from build123d import *

# Parameters (mm, degrees)
SALIENTE_EXTRUIR1_DEPTH    = 172
VACIADO2_T                 = -2
SALIENTE_EXTRUIR2_DEPTH    = 30
CORTAR_EXTRUIR2_DEPTH      = 186.698680663
CORTAR_EXTRUIR2_DEPTH_BACK = 186.698680663
CORTAR_EXTRUIR3_DEPTH      = 184.847763109
CORTAR_EXTRUIR3_DEPTH_BACK = 25
CROQUIS8_R                 = 3.75
CORTAR_EXTRUIR4_DEPTH      = 186.698680663
CORTAR_EXTRUIR4_DEPTH_BACK = 186.698680663
CROQUIS9_W                 = 61.645841287
CROQUIS9_H                 = 31
CORTAR_EXTRUIR5_DEPTH      = 158.419820861
CORTAR_EXTRUIR5_DEPTH_BACK = 158.419820861


with BuildPart() as part:
    # Croquis1 → Saliente-Extruir1 (new body)
    with BuildSketch(Plane(origin=(0, 0, 0), x_dir=(1, 0, 0), z_dir=(0, 1, 0))):
        Polygon((27, 0), (-27, 0), (0, 64.58327957), align=None)
    extrude(amount=SALIENTE_EXTRUIR1_DEPTH)

    # Vaciado2
    vaciado2_openings = [part.faces().sort_by_distance(p)[0] for p in [
        (0, 172, -21.527759857),
    ]]
    offset(amount=VACIADO2_T, openings=vaciado2_openings, kind=Kind.INTERSECTION)

    # Croquis6 → Saliente-Extruir2 (add)
    with BuildSketch(Plane.XZ):
        Polygon((-27, 0), (27, 0), (0, -64.58327957), align=None)
    extrude(amount=SALIENTE_EXTRUIR2_DEPTH)

    # Croquis5 → Cortar-Extruir2 (cut, two sides: drawn at the far end of the back side and taken through both)
    with BuildSketch(Plane(origin=(0, 0, 0), x_dir=(0, 0, -1), z_dir=(1, 0, 0)).offset(-CORTAR_EXTRUIR2_DEPTH_BACK)):
        Polygon((4.522801595, 172), (64.58327957, 172), (64.58327957, 0), align=None)
    extrude(amount=CORTAR_EXTRUIR2_DEPTH + CORTAR_EXTRUIR2_DEPTH_BACK, mode=Mode.SUBTRACT)

    # Croquis8 → Cortar-Extruir3 (cut, two sides: drawn at the far end of the back side and taken through both)
    with BuildSketch(Plane(origin=(0, 2, 0), x_dir=(1, 0, 0), z_dir=(0, 1, 0)).offset(-CORTAR_EXTRUIR3_DEPTH_BACK)):
        with Locations(Location((0, 48.787977385, 0), (0, 0, 270))):
            Circle(CROQUIS8_R)
        with Locations(Location((0, 38.787977385, 0), (0, 0, 270))):
            Circle(CROQUIS8_R)
        with Locations(Location((0, 28.787977385, 0), (0, 0, 270))):
            Circle(CROQUIS8_R)
        with Locations(Location((0, 18.787977385, 0), (0, 0, 270))):
            Circle(CROQUIS8_R)
        with Locations(Location((0, 8.787977385, 0), (0, 0, 270))):
            Circle(CROQUIS8_R)
        with Locations(Location((10, 8.787977385, 0), (0, 0, 270))):
            Circle(CROQUIS8_R)
        with Locations(Location((-10, 8.787977385, 0), (0, 0, 270))):
            Circle(CROQUIS8_R)
        with Locations(Location((10, 18.787977385, 0), (0, 0, 270))):
            Circle(CROQUIS8_R)
        with Locations(Location((-10, 18.787977385, 0), (0, 0, 270))):
            Circle(CROQUIS8_R)
        with Locations(Location((8, 28.787977385, 0), (0, 0, 270))):
            Circle(CROQUIS8_R)
        with Locations(Location((-8, 28.787977385, 0), (0, 0, 270))):
            Circle(CROQUIS8_R)
    extrude(amount=CORTAR_EXTRUIR3_DEPTH + CORTAR_EXTRUIR3_DEPTH_BACK, mode=Mode.SUBTRACT)

    # Croquis9 → Cortar-Extruir4 (cut, two sides: drawn at the far end of the back side and taken through both)
    with BuildSketch(Plane(origin=(0, 0, 0), x_dir=(0, 0, -1), z_dir=(1, 0, 0)).offset(-CORTAR_EXTRUIR4_DEPTH_BACK)):
        with Locations((30.822920644, 156.5)):
            Rectangle(CROQUIS9_W, CROQUIS9_H)
    extrude(amount=CORTAR_EXTRUIR4_DEPTH + CORTAR_EXTRUIR4_DEPTH_BACK, mode=Mode.SUBTRACT)

    # Croquis10 → Cortar-Extruir5 (cut, two sides: drawn at the far end of the back side and taken through both)
    with BuildSketch(Plane(origin=(0, 0, 0), x_dir=(0, 0, -1), z_dir=(1, 0, 0)).offset(-CORTAR_EXTRUIR5_DEPTH_BACK)):
        Polygon((0, 141), (64.58327957, 0), (23.73241025, 141), align=None)
    extrude(amount=CORTAR_EXTRUIR5_DEPTH + CORTAR_EXTRUIR5_DEPTH_BACK, mode=Mode.SUBTRACT)


solid = part.part
Can you work these out from the model? Positions are in its coordinate system, mm. A direction names the side the tool comes from. Give positions to 0.01 mm unless a question says otherwise; leave off trailing zeros. Loops run counter-clockwise (first coordinate to the right, second up) from the corner with the lowest first, then second, coordinate; pieces in that order, holes last. Notation, with made-up numbers: (55.5, 71) - (102.5, 71) arc R26 ccw to (102.5, 94) - close; hole circle Ø11 at (27, 48). An arc over 180 degrees is marked (long way). Return JSON: item names as keys, results as strings.
1. I want a section at A-A on x = -8. Please give me the cut outline in (y, z), and give its area (3 significant figures).
Output values:
{"outline": "(-30, -45.45) - (41.78, -45.45) - (53.1, -40.26) - (2, -40.26) - (2, -32.54) - (-23, -32.54) - (-23, -25.04) - (2, -25.04) - (2, -21.96) - (-23, -21.96) - (-23, -15.62) - (2, -15.62) - (2, -11.96) - (-23, -11.96) - (-23, -5.62) - (2, -5.62) - (2, -2) - (136.63, -2) - (141, 0) - (-30, 0) - close", "area": "1,460 mm²"}
2. If I drill on line 1 (Z direction, x = -8, y = -8); line 2 (Z direction, x = -10, y = -15); line 3 (Z direction, x = -2.5, y = 85.5), over which ranges is the centre line in solid material (lowest first)?
Output values:
{"line 1": "z = -45.45 to -32.54, -25.04 to -21.96, -15.62 to -11.96, -5.62 to 0", "line 2": "z = -40.66 to -31.96, -25.62 to -22.54, -15.04 to -12.54, -5.04 to 0", "line 3": "z = -2 to 0"}
3. I want a section at D-D on y = 50. Please give me the cut outline in (x, z), and give its area (3 significant figures).
Output values:
{"outline": "(-27, 0) - (-9.57, -41.68) - (-7.41, -41.68) - (-24, -2) - (24, -2) - (7.41, -41.68) - (9.57, -41.68) - (27, 0) - close", "area": "278 mm²"}
4. I want a section at C-C on z = -8. Please give me the cut outline in (x, y), and give its area (3 significant figures).
Output values:
{"outline": "(-23.66, -30) - (23.66, -30) - (23.66, 123.53) - (21.49, 123.53) - (21.49, 2) - (13.67, 2) - (13.67, -23) - (6.33, -23) - (6.33, 2) - (3.67, 2) - (3.67, -23) - (-3.67, -23) - (-3.67, 2) - (-6.33, 2) - (-6.33, -23) - (-13.67, -23) - (-13.67, 2) - (-21.49, 2) - (-21.49, 123.53) - (-23.66, 123.53) - close", "area": "1,490 mm²"}
5. We'd pull the mould along X, two halves only. Please class faces 3 (the face through (-10, -23, -19)), 4 (the face through (-2.282, -10.675, -11.764)), 5 (the face through (0, 57, 0)), 6 (the face through (-16.31, 37.7, -25.57)): +X half, -X half, draft (parallel to the pull), parting line (faces both ways), or undercut.
Output values:
{"face 3": "undercut", "face 4": "undercut", "face 5": "draft", "face 6": "-X half"}
6. For faces 1 (the face through (16.69, 37.7, -24.66)), 2 (the face through (1.9, 2, -22.3)), which set-ups out of +Z, -Z, +X, -X, +Y, -Y let a thin tool reach every point of the face, with its end or its side?
Output values:
{"face 1": "-Z, +X, +Y, -Y", "face 2": "+Y"}
7. I want a section at B-B on y = 124. Please give me the cut outline in (x, z).
Output values:
{"outline": "(-27, 0) - (-23.74, -7.79) - (-21.58, -7.79) - (-24, -2) - (24, -2) - (21.58, -7.79) - (23.74, -7.79) - (27, 0) - close"}
8. I'm going to push flat-ended pins straight in: pin 1 Ø3 at (y, z) = (85.5, -26.5) entering from -X; pin 2 Ø6 at (x, z) = (0, -47.5) entering from +Y; pin 3 Ø8 at (x, z) = (-8.5, -49) entering from -Y; pin 4 Ø4 at (x, y) = (-10, 52) entering from -Z. Where does each tip first touch, or does it pass through?
Output values:
{"pin 1": "stops at x = -16.55", "pin 2": "stops at y = 2", "pin 3": "stops at y = -30", "pin 4": "stops at z = -41.66"}
